The model under review builds one solid part; all positions refer to its coordinate system, in mm. Face numbers are marked on the shaded views. A direction names the side the tool comes from. Round coordinates to 2 decimals unless told otherwise and drop trailing zeros. Write each loop counter-clockwise with the first axis right and the second up, starting at its lowest first coordinate (ties: lowest second). Pieces come first, ordered by that corner, then holes. Notation, with made-up numbers: M 34.25,63 L 76.25,63 A18 cw 76.25,69 Z; hole C 64.25,63.5 d7. An arc over 180 degrees is marked long. Write item = value, one per line. Start each with the question number.
Item 1: Take a section at C-C, the plane x = 85. Give the boundary of the cut face in (y, z), plus the area to 3 significant figures.
Item 2: Take a section at B-B, the plane y = -14. Give the boundary of the cut face in (x, z).
Item 3: Take a section at A-A, the plane z = -14.5. Give the boundary of the cut face in (x, y).
Item 4: To check wall thickness, follow line 1 along X through (y, z) = (11, -8.5); line 2 along Y through (x, z) = (108, -3.5); line 3 along X through (y, z) = (-23, -13.5). State the ranges of each line that lie inside material, in increasing order.
Item 5: For pin 1 Ø7 at (y, z) = (11.5, -12.5) entering from +X; pin 2 Ø6 at (x, z) = (53.5, -7.5) entering from -Y; pin 3 Ø12 at (y, z) = (10.5, -5.5) entering from -X, all flat-tipped, find the tip position at first contact; note any pin that passes through.
Item 6: Take a section at D-D, the plane x = -2. Give the boundary of the cut face in (y, z), plus the area to 3 significant figures.
Item 7: The part is to be moulded in two halves that separate along X. For the marked faces 1, 2 and 3, say which applies: +X half, -X half, draft (parallel to the pull), parting line (faces both ways), or undercut.
Item 8: Tool access review of the marked faces 4, 5 and 6: name each direction out of +Z, -Z, +X, -X, +Y, -Y from which nothing blocks a thin tool from reaching the whole face with its end or side.
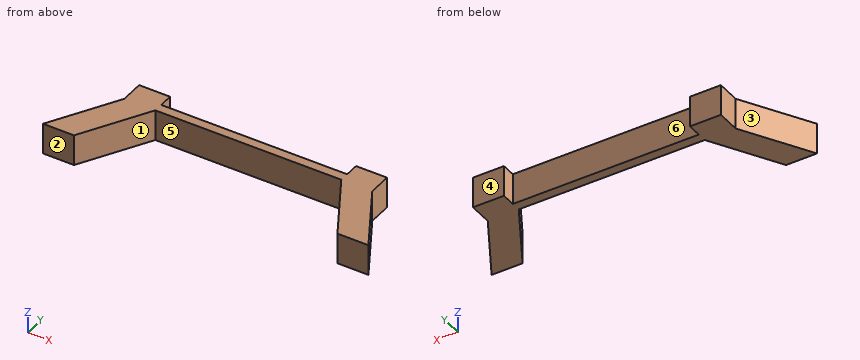
from build123d import *

# Parameters (mm, degrees)
SKETCH_1_W          = 160
SKETCH_1_H          = 20
EXTRUDE_1_DEPTH     = 15
SKETCH_2_W          = 120
SKETCH_2_H          = 20
CUT_EXTRUDE_1_DEPTH = 9
EXTRUDE_2_DEPTH     = 20


with BuildPart() as part:
    # 草图1 → 凸台-拉伸1 (new body)
    with BuildSketch(Plane(origin=(0, 0, 0), x_dir=(1, 0, 0), z_dir=(0, 1, 0))):
        with Locations((80, 10)):
            Rectangle(SKETCH_1_W, SKETCH_1_H)
    extrude(amount=EXTRUDE_1_DEPTH)

    # 草图2 → 切除-拉伸1 (cut)
    with BuildSketch(Plane(origin=(0, 15, 0), x_dir=(1, 0, 0), z_dir=(0, 1, 0))):
        with Locations((80, 10)):
            Rectangle(SKETCH_2_W, SKETCH_2_H)
    extrude(amount=-CUT_EXTRUDE_1_DEPTH, mode=Mode.SUBTRACT)

    # 草图4 → 凸台-拉伸2 (add)
    with BuildSketch(Plane.XY):
        Polygon((0, 0), (-25, -43.301270189), (-5, -43.301270189), (20, 0), align=None)
        Polygon((165, -43.301270189), (140, 0), (160, 0), (185, -43.301270189), align=None)
    extrude(amount=-EXTRUDE_2_DEPTH)


solid = part.part
Response values:
q1.outline = M 0,-20 L 6,-20 L 6,0 L 0,0 Z
q1.area = 120 mm2
q2.outline = M -8.08,-20 L 11.92,-20 L 11.92,0 L -8.08,0 Z; M 148.08,-20 L 168.08,-20 L 168.08,0 L 148.08,0 Z
q3.outline = M -25,-43.3 L -5,-43.3 L 20,0 L 140,0 L 165,-43.3 L 185,-43.3 L 160,0 L 160,15 L 140,15 L 140,6 L 20,6 L 20,15 L 0,15 L 0,0 Z
q4.line_1 = 0 to 20, 140 to 160
q4.line_2 = 0 to 6
q4.line_3 = -13.28 to 6.72, 153.28 to 173.28
q5.pin_1 = 160
q5.pin_2 = 0
q5.pin_3 = 0
q6.outline = M -38.11,-20 L -3.46,-20 L -3.46,0 L -38.11,0 Z
q6.area = 693 mm2
q7.face_1 = undercut
q7.face_2 = draft
q7.face_3 = -X half
q8.face_4 = +Z, -Z, +X, -X, +Y
q8.face_5 = +Z, -Z, -Y
q8.face_6 = +Z, -Z, +Y
